Work out the finished part from the listing and answer in its coordinate system (mm). A direction names the side the tool comes from. Give positions to 0.01 mm unless a question says otherwise; leave off trailing zeros. Use one line per item in the form item = value. Start each with the question number.
from build123d import *

# Parameters (mm, degrees)
SKETCH1_R                    = 9
SKETCH1_R_2                  = 2.6
BOSS_EXTRUDE1_DEPTH          = 36
SKETCH5_W                    = 5
SKETCH5_H                    = 4.08502449
SKETCH5_W_2                  = 8
BOSS_EXTRUDE2_DEPTH          = 22
SKETCH7_W                    = 5
SKETCH7_H                    = 4.653899232
CUT_REVOLVE2_ANGLE           = 90
CUT_REVOLVE2_OTHER_WAY_ANGLE = 90
CIRPATTERN1_COUNT            = 15
SKETCH13_W                   = 5
SKETCH13_H                   = 16.616445935
SKETCH17_R                   = 2
CUT_EXTRUDE1_DEPTH           = 10
BOSS_EXTRUDE3_DEPTH          = 31


with BuildPart() as part:
    # Sketch1 → Boss-Extrude1 (new body)
    with BuildSketch(Plane.XY):
        Circle(SKETCH1_R)
        Circle(SKETCH1_R_2, mode=Mode.SUBTRACT)
    extrude(amount=BOSS_EXTRUDE1_DEPTH)

    # Sketch5 → Cut-Revolve1 (revolve, cut)
    with BuildSketch(Plane(origin=(0, 0, 0), x_dir=(0, 0, -1), z_dir=(1, 0, 0)), mode=Mode.PRIVATE) as cut_revolve1_sk:
        with Locations((-2.5, 6.957487755)):
            Rectangle(SKETCH5_W, SKETCH5_H)
        with Locations((-32, 6.957487755)):
            Rectangle(SKETCH5_W_2, SKETCH5_H)
    revolve(cut_revolve1_sk.sketch.rotate(Axis((0, 0, 0), (0, 0, 1)), 90), axis=Axis((0, 0, 0), (0, 0, 1)), mode=Mode.SUBTRACT)

    # Sketch6 → Boss-Extrude2 (add)
    with BuildSketch(Plane.XY):
        with BuildLine():
            Line((-1, 8.94427191), (-1, 10.94427191))
            ThreePointArc((-1, 10.94427191), (-0.927189817, 11.988569364), (-0.5, 12.94427191))
            Line((-0.5, 12.94427191), (0.5, 12.94427191))
            ThreePointArc((0.5, 12.94427191), (0.927189817, 11.988569364), (1, 10.94427191))
            Line((1, 10.94427191), (1, 8.94427191))
            Line((1, 8.94427191), (-1, 8.94427191))
        make_face()
    boss_extrude2 = extrude(amount=BOSS_EXTRUDE2_DEPTH)

    # Sketch7 → Cut-Revolve2 (revolve, cut)
    with BuildSketch(Plane(origin=(0, 0, 0), x_dir=(0, 0, -1), z_dir=(1, 0, 0))):
        with Locations((-2.5, 11.271221526)):
            Rectangle(SKETCH7_W, SKETCH7_H)
    revolve(axis=Axis((0, 8.94427191, 5), (0, 0, -1)), revolution_arc=CUT_REVOLVE2_ANGLE, mode=Mode.SUBTRACT)

    # Sketch7 → Cut-Revolve2 other way (revolve, cut)
    with BuildSketch(Plane(origin=(0, 0, 0), x_dir=(0, 0, -1), z_dir=(1, 0, 0))):
        with Locations((-2.5, 11.271221526)):
            Rectangle(SKETCH7_W, SKETCH7_H)
    revolve(axis=Axis((0, 8.94427191, 5), (0, 0, 1)), revolution_arc=CUT_REVOLVE2_OTHER_WAY_ANGLE, mode=Mode.SUBTRACT)

    # CirPattern1: Boss-Extrude2 ×15 about axis
    cirpattern1_axis = Axis((0, 0, 0), (0, 0, 1))
    for i in range(1, CIRPATTERN1_COUNT):
        add(boss_extrude2.rotate(cirpattern1_axis, i * 360 / CIRPATTERN1_COUNT))

    # Sketch13 → Cut-Revolve6 (revolve, cut)
    with BuildSketch(Plane(origin=(0, 0, 0), x_dir=(0, 0, -1), z_dir=(1, 0, 0)), mode=Mode.PRIVATE) as cut_revolve6_sk:
        with Locations((-2.5, 8.308222968)):
            Rectangle(SKETCH13_W, SKETCH13_H)
    revolve(cut_revolve6_sk.sketch.rotate(Axis((0, 0, 25.578402878), (0, 0, -1)), 270), axis=Axis((0, 0, 25.578402878), (0, 0, -1)), mode=Mode.SUBTRACT)

    # Sketch17 → Cut-Extrude1 (cut)
    with BuildSketch(Plane(origin=(0, 0, 0), x_dir=(1, 0, 0), z_dir=(0, 1, 0))):
        with Locations(Location((-0.128741976, -25.11123185, 0), (0, 0, 270))):
            Circle(SKETCH17_R)
    extrude(amount=-CUT_EXTRUDE1_DEPTH, mode=Mode.SUBTRACT)

    # Sketch19 → Boss-Extrude3 (add)
    with BuildSketch(Plane.XY.offset(36)):
        Polygon((2.4, 1), (3.9, 1), (3.9, -1), (2.4, -1), (0.9, -1), (0.9, 1), align=None)
    extrude(amount=-BOSS_EXTRUDE3_DEPTH)


solid = part.part
1) Determine the mould class of faces 1 (the flat face through (-1.086, -9.921, 13.381)), 2 (the cylindrical face through (-3.4, -11.5, 13.4)), 3 (the flat face through (3.125, 9.478, 13.381)) for opening direction Y: released by +Y, released by -Y, zero draft, split by the parting line, or undercut.
2) Find the intervals of material crossed by probe 1 along X at (y, z) = (0, 26); probe 2 along Y at (x, z) = (1.75, 17); probe 3 along X at (y, z) = (11.75, 17.5), in increasing order.
3) Flat-ended cylindrical pins translate along their axes: pin 1 Ø0.6 at (y, z) = (10, 13) entering from +X; pin 2 Ø1.7 at (x, y) = (9.5, -5) entering from +Z; pin 3 Ø3 at (x, z) = (-0.13, 25.11) entering from +Y; pin 4 Ø1 at (x, y) = (-0.5, 1.5) entering from +Z. Find the tip coordinate at first contact, or state that the pin passes through.
4) A tool of negligible diameter and unlimited length cuts with its end or side. For faces 4 (the flat face through (1.092, -9.949, 13.381)), 5 (the flat face through (-8.1, -5.83, 13.38)), 6 (the cylindrical face through (-9.52, 7.32, 13.38)), from which of +Z, -Z, +X, -X, +Y, -Y can it reach the whole face along a straight path? Write none if from no direction.
Answer sheet:
q1.face_1 = released by -Y
q1.face_2 = undercut
q1.face_3 = released by +Y
q2.probe_1 = -9 to -2.6, 0.9 to 9
q2.probe_2 = -12.21 to -1.92, -1 to 1, 1.92 to 8.83
q2.probe_3 = -5.43 to -4.43, -0.98 to 0.98, 4.43 to 5.43
q3.pin_1 = 5.66
q3.pin_2 = 22
q3.pin_3 = 9
q3.pin_4 = through
q4.face_4 = +Z, -Z, -Y
q4.face_5 = +Z, -Z
q4.face_6 = +Z, -Z, -X
